from build123d import *

# Parameters (mm, degrees)
F0_W     = 106.479474
F0_H     = 111.292108
F1_DEPTH = 96.52
F2_W     = 99.53875
F2_H     = 182.38613
F3_DEPTH = 181.356
F4_W     = 114.944555
F4_H     = 20.924191
F5_DEPTH = 135.128
F6_R     = 14.283712
F7_DEPTH = 257.302


with BuildPart() as f1:
    # F0 (on Front) → F1 (new body, symmetric)
    with BuildSketch(Plane.XZ):
        Rectangle(F0_W, F0_H)
    extrude(amount=F1_DEPTH, both=True)

    # F2 (on face) → F3 (cut)
    with BuildSketch(Plane.XY.offset(55.646054)):
        Rectangle(F2_W, F2_H)
    extrude(amount=-F3_DEPTH, mode=Mode.SUBTRACT)

    # F4 (on face) → F5 (cut)
    with BuildSketch(Plane.YZ.offset(53.239737)):
        with Locations((-3.193539, 45.183959)):
            Rectangle(F4_W, F4_H)
    extrude(amount=-F5_DEPTH, mode=Mode.SUBTRACT)

    # F6 (on face) → F7 (cut)
    with BuildSketch(Plane.XZ.offset(96.52)):
        with Locations((0, 28.012339)):
            Circle(F6_R)
    extrude(amount=-F7_DEPTH, mode=Mode.SUBTRACT)


solid = f1.part
The model under review builds one solid part; all positions refer to its coordinate system, in mm. A direction names the side the tool comes from. Give positions to 0.01 mm unless a question says otherwise; leave off trailing zeros. Write each loop counter-clockwise with the first axis right and the second up, starting at its lowest first coordinate (ties: lowest second). Pieces come first, ordered by that corner, then holes.
1. Draft analysis for pull direction Z (two halves, no side actions). For faces 3 (the flat face through (-1, -96.52, 1)), 4 (the flat face through (0, 94, 55.646)), 5 (the cylindrical face through (7.679, 93.819, 40.056)), state which applies: +Z half, -Z half, draft (parallel to the pull), parting line (faces both ways), or undercut.
2. Tool access review of faces 1 (the flat face through (-52, 0, -55.646)), 2 (the flat face through (-1, 91.193, 1)): name each direction out of +Z, -Z, +X, -X, +Y, -Y from which nothing blocks a thin tool from reaching the whole face with its end or side.
3. Add section B-B, the plane x = 0. Write out the cut boundary in (y, z), plus the area to 3 significant figures.
4. Add section A-A, the plane x = 45.5. Write out the cut boundary in (y, z), plus the area to 3 significant figures.
5. Add section C-C, the plane y = -36.5. Write out the cut boundary in (x, z), plus the area to 3 significant figures.
6. For P1, Ø3, axis at x = -52, y = -12, coming from the +Z side, flat-tipped, find the tip position at first contact; note if it passes through.
7. Add section D-D, the plane z = 2.5. Write out the cut boundary in (x, y).
8. Wall thickness on L1, parallel to Y at x = 2, z = 45; L2, parallel to X at y = 46, z = -26.5; L3, parallel to Z at x = 0, y = -92.4: over which ranges is each line inside the solid? List them lowest first.
Worked answers:
1. face 3: draft
1. face 4: +Z half
1. face 5: undercut
2. face 1: -Z, +X, -X, +Y, -Y
2. face 2: +Z, -Z
3. outline: (-96.52, -55.65) - (-91.19, -55.65) - (-91.19, 13.73) - (-96.52, 13.73) - close; (-96.52, 42.3) - (-91.19, 42.3) - (-91.19, 55.65) - (-96.52, 55.65) - close; (91.19, -55.65) - (96.52, -55.65) - (96.52, 13.73) - (91.19, 13.73) - close; (91.19, 42.3) - (96.52, 42.3) - (96.52, 55.65) - (91.19, 55.65) - close
3. area: 881 mm2
4. outline: (-96.52, -55.65) - (-91.19, -55.65) - (-91.19, 55.65) - (-96.52, 55.65) - close; (91.19, -55.65) - (96.52, -55.65) - (96.52, 55.65) - (91.19, 55.65) - close
4. area: 1,190 mm2
5. outline: (-53.24, -55.65) - (-49.77, -55.65) - (-49.77, 34.72) - (-53.24, 34.72) - close; (49.77, -55.65) - (53.24, -55.65) - (53.24, 34.72) - (49.77, 34.72) - close
5. area: 627 mm2
6. P1: stops at z = 34.72
7. outline: (-53.24, -96.52) - (53.24, -96.52) - (53.24, 96.52) - (-53.24, 96.52) - close; hole (-49.77, -91.19) - (49.77, -91.19) - (49.77, 91.19) - (-49.77, 91.19) - close
8. L1: y = -96.52 to -91.19, 91.19 to 96.52
8. L2: x = -53.24 to -49.77, 49.77 to 53.24
8. L3: z = -55.65 to 13.73, 42.3 to 55.65
